```python
from build123d import *

# Parameters (mm, degrees)
BASE_FLANGE1_DEPTH           = 5.08
OG_POCKET_DEPTH              = 38.1
SHELL_OF_POCKET_DEPTH        = 38.1
BATTERY_TAIL_HOLE_DEPTH      = 189.182975851
BATTERY_TAIL_HOLE_DEPTH_BACK = 189.182975851
SKETCH11_R                   = 4.064
TAB_BOLT_HOLES_DEPTH         = 189.182975851
SKETCH12_W                   = 30.48
SKETCH12_H                   = 12.716912384
WEIGHT_SAVER_DEPTH           = 10.16
SKETCH13_R                   = 2.286
BOLT_HOLES_THROUGH_DEPTH     = 189.182975851
CUT_EXTRUDE6_DEPTH           = 1.778
POSSIBLE_LIP_R               = 9.144
POSSIBLE_LIP_R_2             = 4.064
BATTERY_LIP_DEPTH            = 6.35


# Sheet-metal steps are written as plain solids
with BuildPart() as part:
    # Sketch1 → Base-Flange1 (new body)
    with BuildSketch(Plane.XY):
        Polygon((0, 0), (46.99, 0), (101.6, 72.558989745), (101.6, 152.4), (-101.6, 152.4), (-101.6, 72.558989745), (-46.99, 0), align=None)
    extrude(amount=-BASE_FLANGE1_DEPTH)

    # Sketch6 → OG Pocket (add)
    with BuildSketch(Plane.XY):
        Polygon((-101.6, 72.558989745), (-101.6, 88.9), (101.6, 88.9), (101.6, 72.558989745), (46.99, 0), (-46.99, 0), align=None)
    extrude(amount=OG_POCKET_DEPTH)

    # Sketch9 → Shell of Pocket (cut)
    with BuildSketch(Plane(origin=(0, 0, -5.08), x_dir=(-1, 0, 0), z_dir=(0, 0, -1))):
        Polygon((-76.889615099, 44.589315736), (-76.889615099, 85.725), (76.889615099, 85.725), (76.889615099, 44.589315736), (45.72, 3.175), (-45.72, 3.175), align=None)
    extrude(amount=-SHELL_OF_POCKET_DEPTH, mode=Mode.SUBTRACT)

    # Sketch10 → Battery Tail Hole (cut, two sides: drawn at the far end of the back side and taken through both)
    with BuildSketch(Plane(origin=(0, 0, -5.08), x_dir=(-1, 0, 0), z_dir=(0, 0, -1)).offset(-BATTERY_TAIL_HOLE_DEPTH_BACK)):
        with BuildLine():
            Line((-5.969, 137.668), (5.969, 137.668))
            ThreePointArc((5.969, 137.668), (13.462, 130.175), (5.969, 122.682))
            Line((5.969, 122.682), (-5.969, 122.682))
            ThreePointArc((-5.969, 122.682), (-13.462, 130.175), (-5.969, 137.668))
        make_face()
    extrude(amount=BATTERY_TAIL_HOLE_DEPTH + BATTERY_TAIL_HOLE_DEPTH_BACK, mode=Mode.SUBTRACT)

    # Sketch11 → Tab Bolt Holes (cut, through all)
    with BuildSketch(Plane(origin=(0, 0, -5.08), x_dir=(-1, 0, 0), z_dir=(0, 0, -1))):
        with Locations((-85.852, 130.175)):
            Circle(SKETCH11_R)
        with Locations((85.852, 130.175)):
            Circle(SKETCH11_R)
    extrude(amount=-TAB_BOLT_HOLES_DEPTH, mode=Mode.SUBTRACT)

    # Sketch12 → Weight Saver (cut)
    with BuildSketch(Plane.ZY.offset(-76.889615099)):
        with Locations((17.78, 79.366543808)):
            Rectangle(SKETCH12_W, SKETCH12_H)
    weight_saver = extrude(amount=-WEIGHT_SAVER_DEPTH, mode=Mode.SUBTRACT)

    # Mirror1: Weight Saver across plane
    add(weight_saver.mirror(Plane(origin=(0, 0, 0), x_dir=(0, 0, 1), z_dir=(1, 0, 0))), mode=Mode.SUBTRACT)

    # Sketch13 → Bolt holes- Through (cut, symmetric)
    with BuildSketch(Plane(origin=(0, 0, -5.08), x_dir=(-1, 0, 0), z_dir=(0, 0, -1))):
        with Locations(Location((-81.885444711, 79.366543808, 0), (0, 0, 90))):
            Circle(SKETCH13_R)
    bolt_holes_through = extrude(amount=BOLT_HOLES_THROUGH_DEPTH, both=True, mode=Mode.SUBTRACT)

    # Mirror2: Bolt holes- Through across plane
    add(bolt_holes_through.mirror(Plane(origin=(0, 0, 0), x_dir=(0, 0, 1), z_dir=(1, 0, 0))), mode=Mode.SUBTRACT)

    # Sketch14 → Cut-Extrude6 (cut)
    with BuildSketch(Plane(origin=(0, 0, -5.08), x_dir=(-1, 0, 0), z_dir=(0, 0, -1))):
        with BuildLine():
            Line((72.263, 152.4), (72.263, 130.175))
            ThreePointArc((72.263, 130.175), (85.852, 116.586), (99.441, 130.175))
            Line((99.441, 130.175), (99.441, 152.4))
            Line((99.441, 152.4), (72.263, 152.4))
        make_face()
    cut_extrude6 = extrude(amount=-CUT_EXTRUDE6_DEPTH, mode=Mode.SUBTRACT)

    # Mirror3: Cut-Extrude6 across plane
    add(cut_extrude6.mirror(Plane(origin=(0, 0, 0), x_dir=(0, 0, 1), z_dir=(1, 0, 0))), mode=Mode.SUBTRACT)

    # Possible Lip → Battery Lip (add)
    # profile 1 of 3: a face of its own
    with BuildSketch(Plane.XY):
        with Locations((85.852, 130.175)):
            Circle(POSSIBLE_LIP_R)
        with Locations(Location((85.852, 130.175, 0), (0, 0, 180))):
            Circle(POSSIBLE_LIP_R_2, mode=Mode.SUBTRACT)
    # profile 2 of 3: a face of its own
    with BuildSketch(Plane.XY):
        with Locations((-85.852, 130.175)):
            Circle(POSSIBLE_LIP_R)
        with Locations(Location((-85.852, 130.175, 0), (0, 0, 180))):
            Circle(POSSIBLE_LIP_R_2, mode=Mode.SUBTRACT)
    # profile 3 of 3: a face of its own
    with BuildSketch(Plane.XY):
        with BuildLine():
            Line((-5.969, 117.602), (5.969, 117.602))
            ThreePointArc((5.969, 117.602), (18.542, 130.175), (5.969, 142.748))
            Line((5.969, 142.748), (-5.969, 142.748))
            ThreePointArc((-5.969, 142.748), (-18.542, 130.175), (-5.969, 117.602))
        make_face()
        with BuildLine():
            Line((-5.969, 122.682), (5.969, 122.682))
            ThreePointArc((5.969, 122.682), (13.462, 130.175), (5.969, 137.668))
            Line((5.969, 137.668), (-5.969, 137.668))
            ThreePointArc((-5.969, 137.668), (-13.462, 130.175), (-5.969, 122.682))
        make_face(mode=Mode.SUBTRACT)
    extrude(amount=BATTERY_LIP_DEPTH)


solid = part.part
```
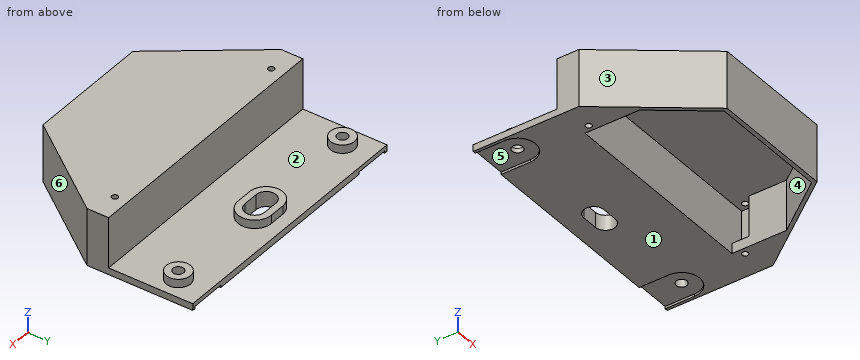
Geometry: final body of the model. Coordinates: model frame, mm. Face numbers are marked on the shaded views. A direction names the side the tool comes from. Give positions to 0.01 mm unless a question says otherwise; leave off trailing zeros. Write each loop counter-clockwise with the first axis right and the second up, starting at its lowest first coordinate (ties: lowest second). Pieces come first, ordered by that corner, then holes.
1. Section query A-A, the plane x = -2. Return loops of the section in (y, z) (3 decimals).
2. Reachability of the marked faces 4, 5 and 6 from +Z, -Z, +X, -X, +Y, -Y: full face, straight path, thin tool, end or side. Return the list, or none.
3. Section query B-B, the plane z = 27. Return loops of the section in (x, y) (3 decimals), then the cut area to 3 significant figures.
4. Section query C-C, the plane x = -43.5. Return loops of the section in (y, z) (3 decimals).
5. Section query D-D, the plane y = 35. Return loops of the section in (x, z).
6. Line query: probe 1 along Y at (x, z) = (-3, 5) (3 decimals); probe 2 along X at (y, z) = (83, 13.5); probe 3 along Y at (x, z) = (28, 20.5) (3 decimals). Output: solid intervals per line, ascending.
7. Pin query (flat end, axial travel): P1, Ø12.5, axis at x = -1, z = -1.5, coming from the -Y side; P2, Ø20, axis at x = -6, y = 129.5, coming from the +Z side; P3, Ø25, axis at x = -38, y = 57.5, coming from the -Z side; P4, Ø10, axis at y = 56, z = 2, coming from the +X side. Return the tip coordinate at first contact, or that it passes through.
8. Draft query along X for the marked faces 1, 2 and 3. Return one class per face: released by +X, released by -X, zero draft, split by the parting line, or undercut.
Computed:
1. outline: (0, -5.08) - (3.175, -5.08) - (3.175, 33.02) - (85.725, 33.02) - (85.725, -5.08) - (122.682, -5.08) - (122.682, 6.35) - (117.602, 6.35) - (117.602, 0) - (88.9, 0) - (88.9, 38.1) - (0, 38.1) - close; (137.668, -5.08) - (152.4, -5.08) - (152.4, 0) - (142.748, 0) - (142.748, 6.35) - (137.668, 6.35) - close
2. face 4: -Z
2. face 5: -Z, +Y
2. face 6: +Z, -Z, +X, -Y
3. outline: (-101.6, 72.559) - (-46.99, 0) - (46.99, 0) - (101.6, 72.559) - (101.6, 88.9) - (-101.6, 88.9) - close; hole (-87.05, 73.008) - (-76.89, 73.008) - (-76.89, 44.589) - (-45.72, 3.175) - (45.72, 3.175) - (76.89, 44.589) - (76.89, 73.008) - (87.05, 73.008) - (87.05, 85.725) - (-87.05, 85.725) - close
3. area: 2,440 mm2
4. outline: (0, -5.08) - (3.175, -5.08) - (3.175, 33.02) - (85.725, 33.02) - (85.725, -5.08) - (152.4, -5.08) - (152.4, 0) - (88.9, 0) - (88.9, 38.1) - (0, 38.1) - close
5. outline: (-73.33, -5.08) - (-69.67, -5.08) - (-69.67, 33.02) - (69.67, 33.02) - (69.67, -5.08) - (73.33, -5.08) - (73.33, 38.1) - (-73.33, 38.1) - close
6. probe 1: y = 0 to 3.175, 85.725 to 88.9, 117.602 to 122.682, 137.668 to 142.748
6. probe 2: x = -101.6 to -87.05, 87.05 to 101.6
6. probe 3: y = 0 to 3.175, 85.725 to 88.9
7. P1: stops at y = 0
7. P2: stops at z = 6.35
7. P3: stops at z = 33.02
7. P4: stops at x = 92.9
8. face 1: zero draft
8. face 2: undercut
8. face 3: released by -X
